Model file for the job. Use its own axes, mm. Face numbers are marked on the shaded views. A direction names the side the tool comes from. Coordinates: 2 decimals unless noted, no trailing zeros. Loops run counter-clockwise (first coordinate to the right, second up) from the corner with the lowest first, then second, coordinate; pieces in that order, holes last.
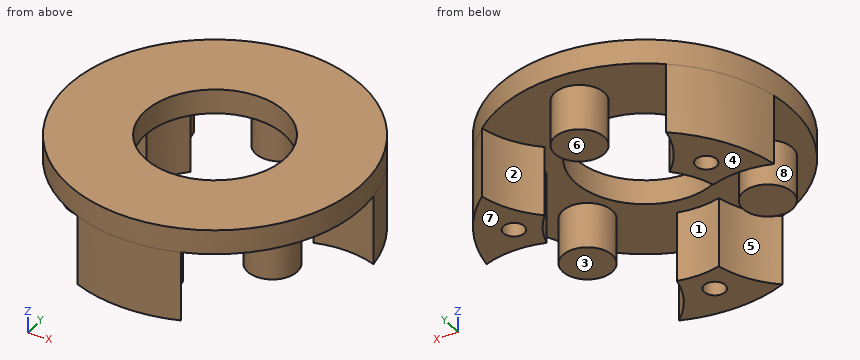
from build123d import *
from build123d.topology import SkipClean

# Parameters (mm, degrees)
SKETCH1_R           = 21
BOSS_EXTRUDE1_DEPTH = 3.5
SKETCH4_R           = 10
CUT_EXTRUDE1_DEPTH  = 8.2
SKETCH11_R          = 1.5
CUT_EXTRUDE2_DEPTH  = 10
BOSS_EXTRUDE2_START = 10
BOSS_EXTRUDE2_DEPTH = 10
SKETCH14_R          = 1.5
CUT_EXTRUDE3_DEPTH  = 5
SKETCH16_R          = 3.55
BOSS_EXTRUDE3_DEPTH = 10


with BuildPart() as part:
    # Sketch1 → Boss-Extrude1 (new body)
    with BuildSketch(Plane.XY):
        Circle(SKETCH1_R)
    extrude(amount=BOSS_EXTRUDE1_DEPTH)

    # Sketch4 → Cut-Extrude1 (cut)
    with BuildSketch(Plane(origin=(0, 0, 0), x_dir=(-1, 0, 0), z_dir=(0, 0, -1))):
        Circle(SKETCH4_R)
    extrude(amount=-CUT_EXTRUDE1_DEPTH, mode=Mode.SUBTRACT)

    # Sketch11 → Cut-Extrude2 (cut)
    with BuildSketch(Plane(origin=(0, 0, 0), x_dir=(-1, 0, 0), z_dir=(0, 0, -1))):
        with Locations((0, 15)):
            Circle(SKETCH11_R)
        with Locations((12.990381057, -7.5)):
            Circle(SKETCH11_R)
        with Locations((-12.990381057, -7.5)):
            Circle(SKETCH11_R)
    extrude(amount=-CUT_EXTRUDE2_DEPTH, mode=Mode.SUBTRACT)

    # Sketch3 → Boss-Extrude2 (add)
    with SkipClean():  # the faces are left unmerged after this step: merging them gives an invalid solid
        with BuildSketch(Plane(origin=(0, 0, 0), x_dir=(-1, 0, 0), z_dir=(0, 0, -1)).offset(BOSS_EXTRUDE2_START)):
            with BuildLine():
                ThreePointArc((-3.021915591, -12.129221993), (-4.618435811, -16.247865366), (-7.4589705, -19.630684121))
                ThreePointArc((-7.4589705, -19.630684121), (0, -21), (7.4589705, -19.630684121))
                ThreePointArc((7.4589705, -19.630684121), (4.618435811, -16.247865366), (3.021915591, -12.129221993))
                ThreePointArc((3.021915591, -12.129221993), (0, -12.5), (-3.021915591, -12.129221993))
            make_face()
            with BuildLine():
                ThreePointArc((-20.730156393, 3.355684121), (-16.38028207, 4.124249945), (-12.01517217, 3.447555327))
                ThreePointArc((-12.01517217, 3.447555327), (-10.825317547, 6.25), (-8.993256579, 8.681666667))
                ThreePointArc((-8.993256579, 8.681666667), (-11.761846259, 12.123615422), (-13.271185893, 16.275))
                ThreePointArc((-13.271185893, 16.275), (-18.186533479, 10.5), (-20.730156393, 3.355684121))
            make_face()
            with BuildLine():
                ThreePointArc((8.993256579, 8.681666667), (10.825317547, 6.25), (12.01517217, 3.447555327))
                ThreePointArc((12.01517217, 3.447555327), (16.38028207, 4.124249945), (20.730156393, 3.355684121))
                ThreePointArc((20.730156393, 3.355684121), (18.186533479, 10.5), (13.271185893, 16.275))
                ThreePointArc((13.271185893, 16.275), (11.761846259, 12.123615422), (8.993256579, 8.681666667))
            make_face()
        extrude(amount=-BOSS_EXTRUDE2_DEPTH)

    # Sketch14 → Cut-Extrude3 (cut)
    with SkipClean():  # the faces are left unmerged after this step: merging them gives an invalid solid
        with BuildSketch(Plane(origin=(0, 0, -10), x_dir=(-1, 0, 0), z_dir=(0, 0, -1))):
            with Locations((13.856406461, 8)):
                Circle(SKETCH14_R)
            with Locations((0, -16)):
                Circle(SKETCH14_R)
            with Locations((-13.856406461, 8)):
                Circle(SKETCH14_R)
        extrude(amount=-CUT_EXTRUDE3_DEPTH, mode=Mode.SUBTRACT)

    # Sketch16 → Boss-Extrude3 (add)
    with SkipClean():  # the faces are left unmerged after this step: merging them gives an invalid solid
        with BuildSketch(Plane.XY.offset(3.5)):
            with Locations((0, 15)):
                Circle(SKETCH16_R)
            with Locations((12.990381057, -7.5)):
                Circle(SKETCH16_R)
            with Locations((-12.990381057, -7.5)):
                Circle(SKETCH16_R)
        extrude(amount=-BOSS_EXTRUDE3_DEPTH)


solid = part.part
Q1. Slice it at C-C (y = 8). List the corners of the cut face in (x, z), and give its area (3 significant figures).
Answers:
outline: (-19.42, -10) - (-15.36, -10) - (-15.36, -5) - (-12.36, -5) - (-12.36, -10) - (-9.6, -10) - (-9.6, 0) - (-6, 0) - (-6, 3.5) - (-19.42, 3.5) - close; (6, 0) - (9.6, 0) - (9.6, -10) - (12.36, -10) - (12.36, -5) - (15.36, -5) - (15.36, -10) - (19.42, -10) - (19.42, 3.5) - (6, 3.5) - close
area: 260 mm2
Q2. Slice it at B-B (x = 0). List the corners of the cut face in (y, z), and give its area (3 significant figures).
Answers:
outline: (-21, -10) - (-17.5, -10) - (-17.5, -5) - (-14.5, -5) - (-14.5, -10) - (-12.5, -10) - (-12.5, 0) - (-10, 0) - (-10, 3.5) - (-21, 3.5) - close; (10, 0) - (11.45, 0) - (11.45, -6.5) - (18.55, -6.5) - (18.55, 0) - (21, 0) - (21, 3.5) - (10, 3.5) - close
area: 193 mm2
Q3. Flat gauge pins, fed straight in: P1, Ø2, axis at x = 12, y = -9, coming from the -Z side; P2, Ø4, axis at x = 16, y = -1, coming from the -Z side; P3, Ø1.5, axis at x = 12.5, z = -7, coming from the -Y side; P4, Ø4, axis at x = 13.86, y = 8, coming from the -Z side. Where does each tip first touch, or does it go through?
Answers:
P1: stops at z = -6.5
P2: stops at z = 0
P3: stops at y = -11.05
P4: stops at z = -10
Q4. Which spindle directions (+Z, -Z, +X, -X, +Y, -Y) get a long thin tool onto all of the face, cutting with end or side? Do the marked faces 1, 2, 3 and 4. Say none if no direction does.
Answers:
face 1: -Z
face 2: -Z, +Y
face 3: -Z, +X, -X, -Y
face 4: -Z, +X, -X, +Y, -Y
Q5. Mould opens along X. For the marked faces 5, 6, 7 and 8 say: +X half, -X half, draft (parallel to the pull), parting line (faces both ways), or undercut.
Answers:
face 5: -X half
face 6: undercut
face 7: draft
face 8: undercut
Q6. Slice it at A-A (z = -6). Count the separate pieces of the cut face and the enclosed holes in it, and give its area (3 significant figures).
Answers:
separate pieces: 6
enclosed holes: 3
area: 345 mm2
Q7. Slice it at D-D (y = 18). List the corners of the cut face in (x, z), and give its area (3 significant figures).
Answers:
outline: (-10.82, 0) - (-1.9, 0) - (-1.9, -6.5) - (1.9, -6.5) - (1.9, 0) - (10.82, 0) - (10.82, 3.5) - (-10.82, 3.5) - close
area: 100 mm2
Q8. Drill centre lines: line 1 (Y direction, x = 0, z = 2.6); line 2 (Z direction, x = -3, y = 13); line 3 (Z direction, x = 14.5, y = -9). Where is each one in solid material? Low to high.
Answers:
line 1: y = -21 to -10, 10 to 21
line 2: z = 0 to 3.5
line 3: z = -6.5 to 3.5
